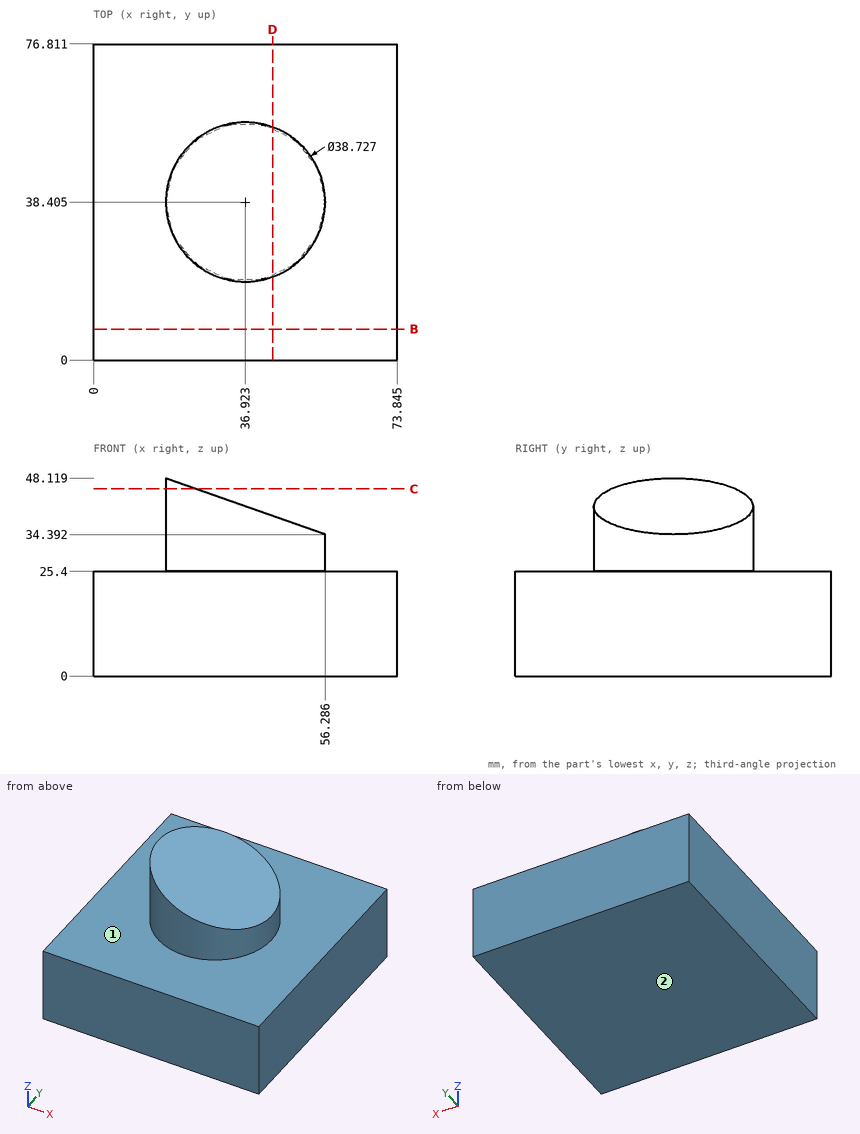
Study the drawing (mm; zero at the part's minimum x, y, z) and answer. A direction names the side the tool comes from. Round coordinates to 2 decimals unless told otherwise and drop trailing zeros. Write each loop counter-clockwise with the first axis right and the second up, starting at its lowest first coordinate (ties: lowest second). Pieces come first, ordered by that corner, then holes.
1) Flat-ended cylindrical pins translate along their axes: P1, Ø5, axis at x = 45, z = 36.5, coming from the -Y side; P2, Ø5, axis at y = 55, z = 36.5, coming from the +X side. Find the tip coordinate at first contact, or state that the pin passes through.
2) Which of the six approach directions +Z, -Z, +X, -X, +Y, -Y give full straight-line access (tool end or side, diameter ignored) to the marked faces 1 and 2?
3) A cutting plane is placed at C-C on z = 45.5. Determine the outline of the cut face in (x, y) (1 decimal), and give its area (3 significant figures).
4) A cutting plane is placed at B-B on y = 7.5. Determine the outline of the cut face in (x, z) (1 decimal).
5) A cutting plane is placed at D-D on x = 43.5. Determine the outline of the cut face in (y, z).
6) Consider probe 1 along Z at (x, y) = (7.5, 33); probe 2 along Y at (x, z) = (51.5, 36); probe 3 along Z at (x, y) = (35.5, 46). Determine where each line is inside the solid, lowest interval first.
Entries:
1. P1: stops at y = 19.86
1. P2: stops at x = 50.2
2. face 1: +Z
2. face 2: -Z, +X, -X, +Y, -Y
3. outline: (24.9, 23.2) - (24.9, 53.6) arc R19.4 ccw to start
3. area: 157 mm2
4. outline: (0, 0) - (73.8, 0) - (73.8, 25.4) - (0, 25.4) - close
5. outline: (0, 0) - (76.81, 0) - (76.81, 25.4) - (56.62, 25.4) - (56.62, 38.92) - (20.19, 38.92) - (20.19, 25.4) - (0, 25.4) - close
6. probe 1: z = 0 to 25.4
6. probe 2: y = 25.66 to 51.15
6. probe 3: z = 0 to 41.76
